Geometry: final body of the model. Coordinates: model frame, mm. Round coordinates to 2 decimals unless told otherwise and drop trailing zeros. Order: outer loops, then holes, each group sorted by start corner. A loop starts at its lowest first (then second) coordinate and runs counter-clockwise, first axis right, second up. Notation, with made-up numbers: (71, 18) - (108, 18) arc R31 ccw to (108, 47) - close; hole circle Ø3 at (27, 11). An arc over 180 degrees is marked (long way). Put each result on its own line as item: value. Start each with the question number.
(1) Section D-D (x = 1). Output: boundary loops of the cut face in (y, z).
(2) Pin query (flat end, axial travel): P1, Ø10, axis at x = -10.5, y = -9.5, coming from the -Z side. Return the tip coordinate at first contact, or that it passes through.
(3) Section B-B (y = -10). Output: boundary loops of the cut face in (x, z).
(4) Material intervals for L1, parallel to X at y = -2.75, z = 9.5; L2, parallel to X at y = -13.5, z = 17.5; L3, parallel to Z at x = 142.5, y = -1.75, sorted ascending. Write a range as [from, to].
(5) Section A-A (z = 39). Output: boundary loops of the cut face in (x, y), and give its area (3 significant figures).
(6) Section C-C (z = 18). Output: boundary loops of the cut face in (x, y).
from build123d import *

# Parameters (mm, degrees)
F1_DEPTH = 19.05
F2_DEPTH = 19.05


with BuildPart() as f1:
    # F0 (on Front) → F1 (new body)
    with BuildSketch(Plane.XZ):
        with BuildLine():
            Line((171.029483, 0), (196.429483, 0))
            Line((196.429483, 0), (196.429483, 125.8062))
            Line((196.429483, 125.8062), (171.029483, 125.8062))
            Line((171.029483, 125.8062), (-53.227117, 125.8062))
            Line((-53.227117, 125.8062), (-78.627117, 125.8062))
            Line((-78.627117, 125.8062), (-78.627117, 0))
            Line((-78.627117, 0), (-53.227117, 0))
            ThreePointArc((-53.227117, 0), (58.901183, 47.101938), (171.029483, 0))
        make_face()
        with BuildLine():
            Line((69.962883, 0), (171.029483, 0))
            ThreePointArc((171.029483, 0), (58.901183, 47.101938), (-53.227117, 0))
            Line((-53.227117, 0), (69.962883, 0))
        make_face()
    extrude(amount=F1_DEPTH)

    # F0 (on Front) → F2 (cut)
    with BuildSketch(Plane.XZ):
        with BuildLine():
            Line((69.962883, 0), (171.029483, 0))
            ThreePointArc((171.029483, 0), (58.901183, 47.101938), (-53.227117, 0))
            Line((-53.227117, 0), (69.962883, 0))
        make_face()
    extrude(amount=F2_DEPTH, mode=Mode.SUBTRACT)


solid = f1.part
Checks:
1. outline: (-19.05, 36.04) - (0, 36.04) - (0, 125.81) - (-19.05, 125.81) - close
2. P1: stops at z = 28.36
3. outline: (-78.63, 0) - (-53.23, 0) arc R157.01 cw to (171.03, 0) - (196.43, 0) - (196.43, 125.81) - (-78.63, 125.81) - close
4. L1: x = [-78.63, -43.05], [160.85, 196.43]
4. L2: x = [-78.63, -32.86], [150.66, 196.43]
4. L3: z = [23, 125.81]
5. outline: (-78.63, -19.05) - (9.12, -19.05) - (9.12, 0) - (-78.63, 0) - close; (108.69, -19.05) - (196.43, -19.05) - (196.43, 0) - (108.69, 0) - close
5. area: 3,340 mm²
6. outline: (-78.63, -19.05) - (-32.16, -19.05) - (-32.16, 0) - (-78.63, 0) - close; (149.96, -19.05) - (196.43, -19.05) - (196.43, 0) - (149.96, 0) - close
